```python
from build123d import *

# Parameters (mm, degrees)
F1_DEPTH = 3
F3_DEPTH = 38
F5_DEPTH = 5
F7_DEPTH = 10
F9_DEPTH = 67.701


# Not quite as in the source:
# - a feature names something its author has since deleted; it is built from what else it names


with BuildPart() as f1:
    # F0 (on Top) → F1 (new body)
    with BuildSketch(Plane.XY):
        with BuildLine():
            Line((-25.35, -36.5), (25.35, -36.5))
            ThreePointArc((25.35, -36.5), (31.3604076401, -34.0104076401), (33.85, -28))
            Line((33.85, -28), (33.85, 28))
            ThreePointArc((33.85, 28), (31.3604076401, 34.0104076401), (25.35, 36.5))
            Line((25.35, 36.5), (-25.35, 36.5))
            ThreePointArc((-25.35, 36.5), (-31.3604076401, 34.0104076401), (-33.85, 28))
            Line((-33.85, 28), (-33.85, -28))
            ThreePointArc((-33.85, -28), (-31.3604076401, -34.0104076401), (-25.35, -36.5))
        make_face()
    extrude(amount=F1_DEPTH)

    # F2 (on face) → F3 (join)
    with BuildSketch(Plane.XY.offset(3)):
        with BuildLine():
            ThreePointArc((-25.35, 36.5), (-31.3604076401, 34.0104076401), (-33.85, 28))
            Line((-33.85, 28), (-33.85, -28))
            ThreePointArc((-33.85, -28), (-31.3604076401, -34.0104076401), (-25.35, -36.5))
            Line((-25.35, -36.5), (25.35, -36.5))
            ThreePointArc((25.35, -36.5), (31.3604076401, -34.0104076401), (33.85, -28))
            Line((33.85, -28), (33.85, 28))
            ThreePointArc((33.85, 28), (31.3604076401, 34.0104076401), (25.35, 36.5))
            Line((25.35, 36.5), (-25.35, 36.5))
        make_face()
        with BuildLine():
            ThreePointArc((30.35, -27), (28.5926406871, -31.2426406871), (24.35, -33))
            Line((24.35, -33), (-24.35, -33))
            ThreePointArc((-24.35, -33), (-28.5926406871, -31.2426406871), (-30.35, -27))
            Line((-30.35, -27), (-30.35, 27))
            ThreePointArc((-30.35, 27), (-28.5926406871, 31.2426406871), (-24.35, 33))
            Line((-24.35, 33), (24.35, 33))
            ThreePointArc((24.35, 33), (28.5926406871, 31.2426406871), (30.35, 27))
            Line((30.35, 27), (30.35, -27))
        make_face(mode=Mode.SUBTRACT)
    extrude(amount=F3_DEPTH)

    # F4 (on face) → F5 (join)
    with BuildSketch(Plane.XY.offset(41)):
        with BuildLine():
            Line((25.35, 36.5), (-25.35, 36.5))
            ThreePointArc((-25.35, 36.5), (-31.3604076401, 34.0104076401), (-33.85, 28))
            Line((-33.85, 28), (-33.85, -28))
            ThreePointArc((-33.85, -28), (-31.3604076401, -34.0104076401), (-25.35, -36.5))
            Line((-25.35, -36.5), (25.35, -36.5))
            ThreePointArc((25.35, -36.5), (31.3604076401, -34.0104076401), (33.85, -28))
            Line((33.85, -28), (33.85, 28))
            ThreePointArc((33.85, 28), (31.3604076401, 34.0104076401), (25.35, 36.5))
        make_face()
        Polygon((24.35, 33), (30.35, 33), (30.35, 27), (30.35, 12), (30.35, -12), (30.35, -27), (30.35, -33), (24.35, -33), (9.35, -33), (-9.35, -33), (-24.35, -33), (-30.35, -33), (-30.35, -27), (-30.35, -12), (-30.35, 12), (-30.35, 27), (-30.35, 33), (-24.35, 33), (-9.35, 33), (9.35, 33), align=None, mode=Mode.SUBTRACT)
        with BuildLine():
            ThreePointArc((-30.35, 27), (-28.5926406871, 31.2426406871), (-24.35, 33))
            Line((-24.35, 33), (-30.35, 33))
            Line((-30.35, 33), (-30.35, 27))
        make_face()
        with BuildLine():
            Line((30.35, 27), (30.35, 33))
            Line((30.35, 33), (24.35, 33))
            ThreePointArc((24.35, 33), (28.5926406871, 31.2426406871), (30.35, 27))
        make_face()
        with BuildLine():
            Line((30.35, -33), (30.35, -27))
            ThreePointArc((30.35, -27), (28.5926406871, -31.2426406871), (24.35, -33))
            Line((24.35, -33), (30.35, -33))
        make_face()
        with BuildLine():
            ThreePointArc((-24.35, -33), (-28.5926406871, -31.2426406871), (-30.35, -27))
            Line((-30.35, -27), (-30.35, -33))
            Line((-30.35, -33), (-24.35, -33))
        make_face()
        with BuildLine():
            Line((30.35, -27), (30.35, -12))
            Line((30.35, -12), (9.35, -33))
            Line((9.35, -33), (24.35, -33))
            ThreePointArc((24.35, -33), (28.5926406871, -31.2426406871), (30.35, -27))
        make_face()
        with BuildLine():
            ThreePointArc((30.35, 27), (28.5926406871, 31.2426406871), (24.35, 33))
            Line((24.35, 33), (9.35, 33))
            Line((9.35, 33), (30.35, 12))
            Line((30.35, 12), (30.35, 27))
        make_face()
        with BuildLine():
            Line((-30.35, 12), (-9.35, 33))
            Line((-9.35, 33), (-24.35, 33))
            ThreePointArc((-24.35, 33), (-28.5926406871, 31.2426406871), (-30.35, 27))
            Line((-30.35, 27), (-30.35, 12))
        make_face()
        with BuildLine():
            Line((-9.35, -33), (-30.35, -12))
            Line((-30.35, -12), (-30.35, -27))
            ThreePointArc((-30.35, -27), (-28.5926406871, -31.2426406871), (-24.35, -33))
            Line((-24.35, -33), (-9.35, -33))
        make_face()
    extrude(amount=-F5_DEPTH)

    # F6 (on face) → F7 (join)
    with BuildSketch(Plane.XY.offset(41)):
        with BuildLine():
            Line((25.35, 36.5), (-25.35, 36.5))
            ThreePointArc((-25.35, 36.5), (-31.3604076401, 34.0104076401), (-33.85, 28))
            Line((-33.85, 28), (-33.85, -28))
            ThreePointArc((-33.85, -28), (-31.3604076401, -34.0104076401), (-25.35, -36.5))
            Line((-25.35, -36.5), (25.35, -36.5))
            ThreePointArc((25.35, -36.5), (31.3604076401, -34.0104076401), (33.85, -28))
            Line((33.85, -28), (33.85, 28))
            ThreePointArc((33.85, 28), (31.3604076401, 34.0104076401), (25.35, 36.5))
        make_face()
        with BuildLine():
            Line((9.35, 33), (24.35, 33))
            ThreePointArc((24.35, 33), (28.5926406871, 31.2426406871), (30.35, 27))
            Line((30.35, 27), (30.35, 12))
            Line((30.35, 12), (30.35, -12))
            Line((30.35, -12), (30.35, -27))
            ThreePointArc((30.35, -27), (28.5926406871, -31.2426406871), (24.35, -33))
            Line((24.35, -33), (9.35, -33))
            Line((9.35, -33), (-9.35, -33))
            Line((-9.35, -33), (-24.35, -33))
            ThreePointArc((-24.35, -33), (-28.5926406871, -31.2426406871), (-30.35, -27))
            Line((-30.35, -27), (-30.35, -12))
            Line((-30.35, -12), (-30.35, 12))
            Line((-30.35, 12), (-30.35, 27))
            ThreePointArc((-30.35, 27), (-28.5926406871, 31.2426406871), (-24.35, 33))
            Line((-24.35, 33), (-9.35, 33))
            Line((-9.35, 33), (9.35, 33))
        make_face(mode=Mode.SUBTRACT)
    extrude(amount=F7_DEPTH)

    # F8 (on face) → F9 (cut, through all)
    with BuildSketch(Plane.YZ.offset(33.85)):
        with BuildLine():
            Line((-1, 0), (1, 0))
            ThreePointArc((1, 0), (0, 1), (-1, 0))
        make_face()
    extrude(amount=-F9_DEPTH, mode=Mode.SUBTRACT)


solid = f1.part
```
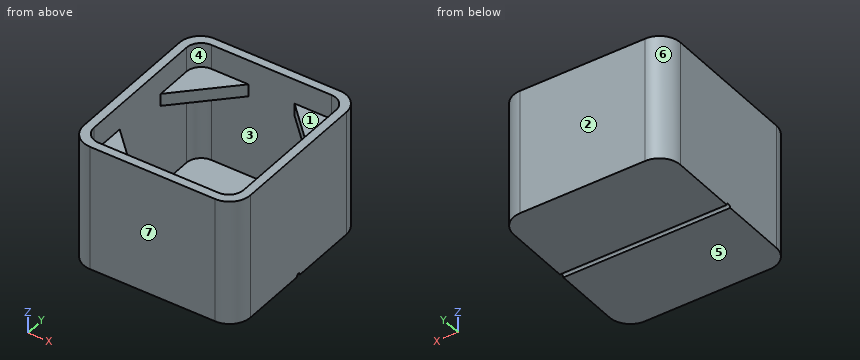
Could you check a few things on this model? Use its own coordinates, in mm. Face numbers are marked on the shaded views. A direction names the side the tool comes from. Give positions to 0.01 mm unless a question says otherwise; leave off trailing zeros. Write each loop counter-clockwise with the first axis right and the second up, starting at its lowest first coordinate (ties: lowest second). Pieces come first, ordered by that corner, then holes. Notation, with made-up numbers: (-35, 8) -> (-6, 8) arc R27 ccw to (-6, 33) -> close; hole circle Ø8 at (46, -15). An arc over 180 degrees is marked (long way). Write each question's results on one line, items separated by ' | '.
1. On a 3-axis mill with a long thin cutter (end or side, diameter ignored), from which of +Z, -Z, +X, -X, +Y, -Y can I reach the whole of each face in a straight line? I mean the marked faces 1, 2 and 3. Say none if no direction works.
Check sheet entries:
face 1: +Z | face 2: +Z, -Z, +X, -X, +Y | face 3: none
2. I need wall thicknesses on L1, parallel to X at y = 18.5, z = 15; L2, parallel to Y at x = 2.5, z = 44.5; L3, parallel to Z at x = 26, y = -29. Which ranges of each line are inside material? Lowest first, please.
Check sheet entries:
L1: x = -33.85 to -30.35, 30.35 to 33.85 | L2: y = -36.5 to -33, 33 to 36.5 | L3: z = 0 to 3, 36 to 41
3. I want a section at B-B, the plane x = 11.5. Write out the boundary of the cut face in (y, z).
Check sheet entries:
outline: (-36.5, 0) -> (-1, 0) arc R1 cw to (1, 0) -> (36.5, 0) -> (36.5, 51) -> (33, 51) -> (33, 41) -> (30.85, 41) -> (30.85, 36) -> (33, 36) -> (33, 3) -> (-33, 3) -> (-33, 36) -> (-30.85, 36) -> (-30.85, 41) -> (-33, 41) -> (-33, 51) -> (-36.5, 51) -> close
4. If we mould it in two halves opening along Y, with no side actions, what happens to the marked faces 4, 5, 6 and 7? For each: released by +Y, released by -Y, zero draft, split by the parting line, or undercut.
Check sheet entries:
face 4: undercut | face 5: zero draft | face 6: released by +Y | face 7: released by -Y
5. I want a section at D-D, the plane x = -18. Write out the boundary of the cut face in (y, z), then the cut area to 3 significant figures.
Check sheet entries:
outline: (-36.5, 0) -> (-1, 0) arc R1 cw to (1, 0) -> (36.5, 0) -> (36.5, 51) -> (33, 51) -> (33, 41) -> (24.35, 41) -> (24.35, 36) -> (33, 36) -> (33, 3) -> (-33, 3) -> (-33, 36) -> (-24.35, 36) -> (-24.35, 41) -> (-33, 41) -> (-33, 51) -> (-36.5, 51) -> close | area: 640 mm²
6. Will these pins go through, and if not, where does the flat tip stop? pin 1 Ø10.5 at (x, y) = (21, 21.5) entering from +Z; pin 2 Ø6 at (x, y) = (4.5, 23.5) entering from +Z.
Check sheet entries:
pin 1: stops at z = 41 | pin 2: stops at z = 3
7. I want a section at C-C, the plane z = 48. Write out the boundary of the cut face in (x, y).
Check sheet entries:
outline: (-33.85, -28) arc R8.5 ccw to (-25.35, -36.5) -> (25.35, -36.5) arc R8.5 ccw to (33.85, -28) -> (33.85, 28) arc R8.5 ccw to (25.35, 36.5) -> (-25.35, 36.5) arc R8.5 ccw to (-33.85, 28) -> close; hole (-30.35, -27) arc R6 ccw to (-24.35, -33) -> (24.35, -33) arc R6 ccw to (30.35, -27) -> (30.35, 27) arc R6 ccw to (24.35, 33) -> (-24.35, 33) arc R6 ccw to (-30.35, 27) -> close
8. I want a section at A-A, the plane y = 0. Write out the boundary of the cut face in (x, z), then the cut area to 3 significant figures.
Check sheet entries:
outline: (-33.85, 1) -> (33.85, 1) -> (33.85, 51) -> (30.35, 51) -> (30.35, 3) -> (-30.35, 3) -> (-30.35, 51) -> (-33.85, 51) -> close | area: 471 mm²
